CAD build for the part. Positions are in the model's coordinates, mm. Round coordinates to 2 decimals unless told otherwise and drop trailing zeros. Write each loop counter-clockwise with the first axis right and the second up, starting at its lowest first coordinate (ties: lowest second). Pieces come first, ordered by that corner, then holes. Notation, with made-up numbers: (65.25, 59.25) -> (112.25, 59.25) arc R13 cw to (112.25, 63.25) -> close; hole circle Ø10 at (80.5, -16). An arc over 180 degrees is marked (long way). Put each result on its own line as item: value. Start each with the question number.
1. Drill centre lines: line 1 (X direction, y = 407.5, z = 4); line 2 (Y direction, x = -10, z = 6); line 3 (X direction, y = 430, z = 3.25). Where is each one in solid material? Low to high. Write a range as from..to.
2. Saw through at B-B on x = -399. List the corners of the cut face in (y, z).
3. Flat gauge pins, fed straight in: P1, Ø5.5, axis at x = -607.5, y = 10, coming from the -Z side; P2, Ø9.5, axis at x = -630, y = 407.5, coming from the +Z side. Where does each tip first touch, or does it go through?
4. Saw through at C-C on z = 1.75. State how many separate pieces and enclosed holes the cut face has, and give its area (3 significant figures).
5. Saw through at A-A on y = 146. List the corners of the cut face in (x, z), and give its area (3 significant figures).
from build123d import *

# Parameters (mm, degrees)
ESQUISSE1_W             = 640
ESQUISSE1_H             = 440
ESQUISSE1_W_2           = 600
ESQUISSE1_H_2           = 400
BOSS_EXTRU_1_DEPTH      = 10
ESQUISSE2_R             = 3
ENL_V_MAT_EXTRU_1_DEPTH = 11


with BuildPart() as part:
    # Esquisse1 → Boss.-Extru.1 (new body)
    with BuildSketch(Plane.XY):
        with Locations((-320, 220)):
            Rectangle(ESQUISSE1_W, ESQUISSE1_H)
        with Locations((-320, 220)):
            Rectangle(ESQUISSE1_W_2, ESQUISSE1_H_2, mode=Mode.SUBTRACT)
    extrude(amount=BOSS_EXTRU_1_DEPTH)

    # Esquisse2 → Enlèv. mat.-Extru.1 (cut, through all)
    with BuildSketch(Plane.XY.offset(10)):
        with Locations((-32.5, 430)):
            Circle(ESQUISSE2_R)
        with Locations((-10, 407.5)):
            Circle(ESQUISSE2_R)
        with Locations((-607.5, 430)):
            Circle(ESQUISSE2_R)
        with Locations((-630, 407.5)):
            Circle(ESQUISSE2_R)
        with Locations((-630, 32.5)):
            Circle(ESQUISSE2_R)
        with Locations((-607.5, 10)):
            Circle(ESQUISSE2_R)
        with Locations((-32.5, 10)):
            Circle(ESQUISSE2_R)
        with Locations((-10, 32.5)):
            Circle(ESQUISSE2_R)
    extrude(amount=-ENL_V_MAT_EXTRU_1_DEPTH, mode=Mode.SUBTRACT)


solid = part.part
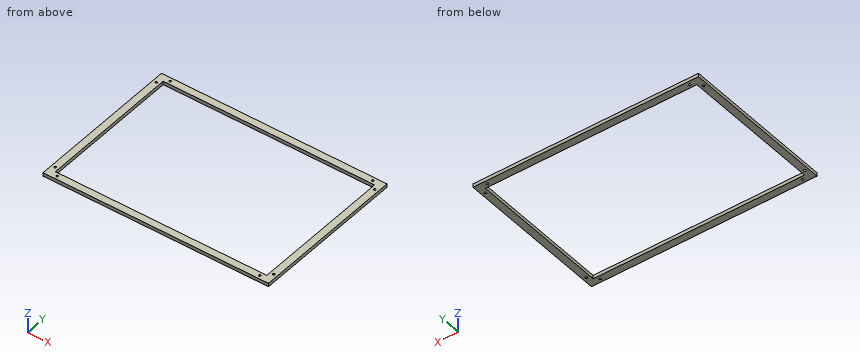
Return value:
1. line 1: x = -640..-633, -627..-620, -20..-13, -7..0
1. line 2: y = 0..29.5, 35.5..404.5, 410.5..440
1. line 3: x = -640..-610.5, -604.5..-35.5, -29.5..0
2. outline: (0, 0) -> (20, 0) -> (20, 10) -> (0, 10) -> close; (420, 0) -> (440, 0) -> (440, 10) -> (420, 10) -> close
3. P1: passes through
3. P2: stops at z = 10
4. separate pieces: 1
4. enclosed holes: 9
4. area: 41,400 mm^2
5. outline: (-640, 0) -> (-620, 0) -> (-620, 10) -> (-640, 10) -> close; (-20, 0) -> (0, 0) -> (0, 10) -> (-20, 10) -> close
5. area: 400 mm^2
